The figure shows three views and two pictorial views of one solid part (mm, origin at its lowest corner). Answer the questions. A direction names the side the tool comes from. Give positions to 0.01 mm unless a question says otherwise; leave off trailing zeros. Loops run counter-clockwise (first coordinate to the right, second up) from the corner with the lowest first, then second, coordinate; pieces in that order, holes last. Notation, with made-up numbers: (3, 14.5) - (19, 14.5) arc R23 ccw to (19, 27.5) - close; hole circle Ø2 at (7.25, 44). An arc over 180 degrees is marked (long way). Write each question's results on one line, items separated by ' | '.
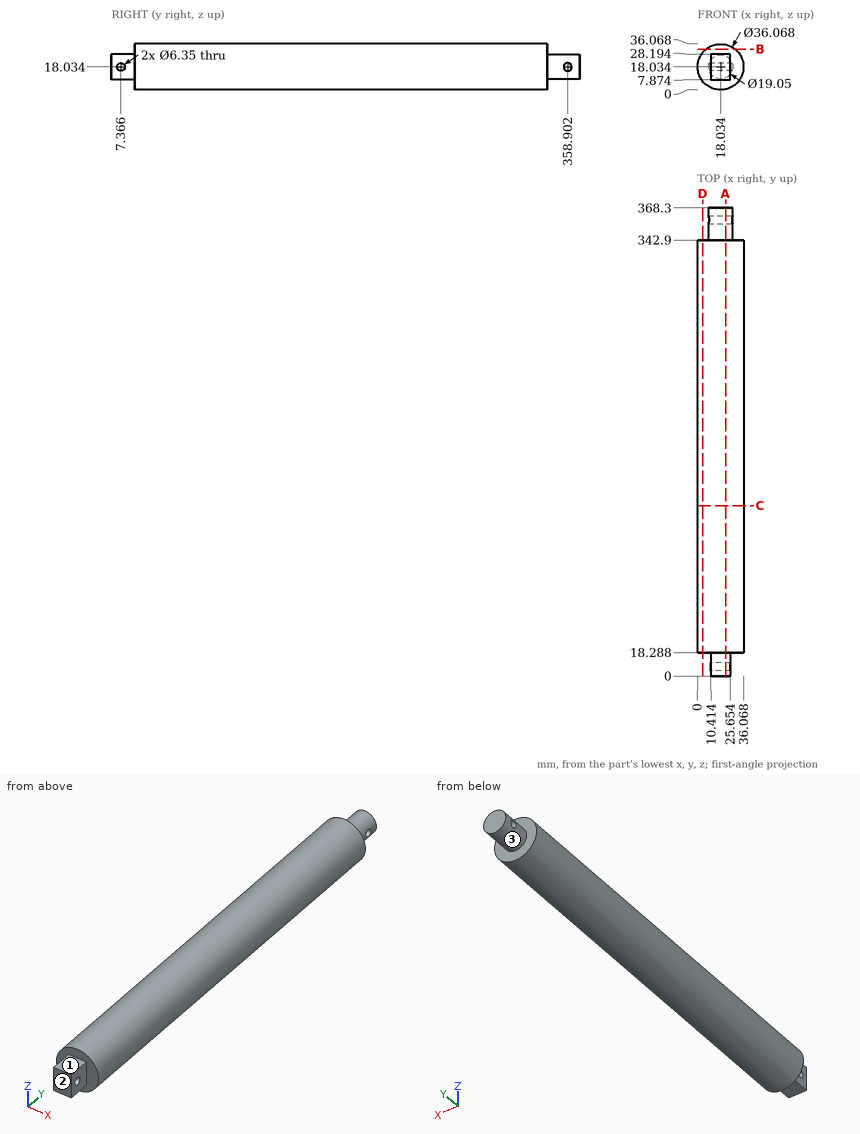
Item 1: A cutting plane is placed at B-B, the plane z = 32. Determine the outline of the cut face in (x, y), plus the area to 3 significant figures.
Values found:
outline: (6.62, 18.29) - (29.44, 18.29) - (29.44, 342.9) - (6.62, 342.9) - close | area: 7,410 mm²
Item 2: Flat-ended cylindrical pins translate along their axes: P1, Ø5, axis at x = 5, y = 209, coming from the +Z side; P2, Ø10, axis at x = 10, z = 4.5, coming from the -Y side; P3, Ø8.5, axis at y = 358.902, z = 18.034, coming from the +X side; P4, Ø8.5, axis at y = 7.366, z = 18.034, coming from the +X side. Find the tip coordinate at first contact, or state that the pin passes through.
Values found:
P1: stops at z = 32.67 | P2: stops at y = 0 | P3: stops at x = 27.56 | P4: stops at x = 25.65
Item 3: A cutting plane is placed at C-C, the plane y = 134. Determine the outline of the cut face in (x, z), plus the area to 3 significant figures.
Values found:
outline: circle Ø36.07 at (18.03, 18.03) | area: 1,020 mm²
Item 4: For the marked faces 1, 2 and 3, determine the directions among +Z, -Z, +X, -X, +Y, -Y from which every point of the face is accessible in a straight line to the end or side of a thin tool.
Values found:
face 1: +Z, +X, -X, -Y | face 2: +Z, -Z, +X, -X, -Y | face 3: +Y
Item 5: A cutting plane is placed at A-A, the plane x = 22. Count the separate pieces of the cut face and the enclosed holes in it, plus the area to 3 significant figures.
Values found:
separate pieces: 1 | enclosed holes: 2 | area: 12,200 mm²
Item 6: A cutting plane is placed at D-D, the plane x = 4. Determine the outline of the cut face in (y, z), plus the area to 3 significant figures.
Values found:
outline: (18.29, 6.71) - (342.9, 6.71) - (342.9, 29.36) - (18.29, 29.36) - close | area: 7,350 mm²
Item 7: Find the intervals of material crossed by line 1 along Y through (x, z) = (15, 29); line 2 along Y through (x, z) = (15, 20.5); line 3 along Y through (x, z) = (23, 16.5), in increasing order. Write a range as [from, to].
Values found:
line 1: y = [18.29, 342.9] | line 2: y = [0, 5.37], [9.37, 356.9], [360.9, 368.3] | line 3: y = [0, 4.59], [10.15, 356.12], [361.68, 368.3]
